Here's how the part is built. I have some questions about the finished solid (model axes, mm). Face numbers are marked on the shaded views. Coordinates: 2 decimals unless noted, no trailing zeros. Write each loop counter-clockwise with the first axis right and the second up, starting at its lowest first coordinate (ties: lowest second). Pieces come first, ordered by that corner, then holes. Notation, with made-up numbers: (64.5, -25) -> (74.5, -25) arc R28 ccw to (74.5, 8) -> close; hole circle Ø7 at (31.25, 34.25). An arc over 180 degrees is marked (long way). Use a Markdown table: item, result. Add a question column.
Item 1: If I drill on line 1 along Y through (x, z) = (0, 87); line 2 along X through (y, z) = (28.5, 110.5); line 3 along Y through (x, z) = (50, 68.5), over which ranges is the centre line in solid material (lowest first)? Write a range as from..to.
Item 2: Imagine slicing it at A-A, the plane x = 0. Write out the boundary of the cut face in (y, z) (3 decimals), and give its area (3 significant figures).
Item 3: Imagine slicing it at D-D, the plane z = 12.5. Write out the boundary of the cut face in (x, y).
Item 4: Will these pins go through, and if not, where does the flat tip stop? pin 1 Ø1.5 at (y, z) = (8.5, 82.5) entering from +X; pin 2 Ø10 at (y, z) = (50.5, 102.5) entering from +X; pin 3 Ø5 at (y, z) = (-76.5, 115.5) entering from +X.
Item 5: Imagine slicing it at C-C, the plane z = 143. Write out the boundary of the cut face in (x, y).
Item 6: If we mould it in two halves opening along X, with no side actions, what happens to the marked faces 1, 2 and 3? For each: pulls with the +X half, pulls with the -X half, needs draft (parallel to the pull), parting line crosses it, or undercut.
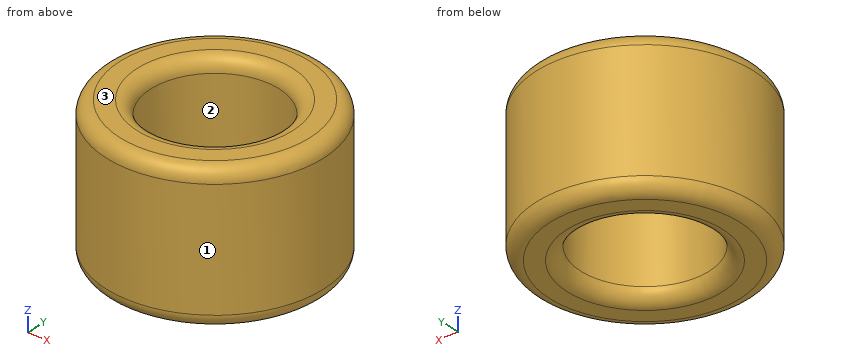
```python
from build123d import *

# Parameters (mm, degrees)
SKETCH1_R           = 127
BOSS_EXTRUDE1_DEPTH = 170
SKETCH2_R           = 75
CUT_EXTRUDE1_DEPTH  = 171
FILLET1_R           = 15.875


with BuildPart() as part:
    # Sketch1 → Boss-Extrude1 (new body)
    with BuildSketch(Plane.XY):
        Circle(SKETCH1_R)
    extrude(amount=BOSS_EXTRUDE1_DEPTH)

    # Sketch2 → Cut-Extrude1 (cut, through all)
    with BuildSketch(Plane.XY.offset(170)):
        Circle(SKETCH2_R)
    extrude(amount=-CUT_EXTRUDE1_DEPTH, mode=Mode.SUBTRACT)

    # Fillet1
    fillet1_edges = [part.edges().sort_by_distance(p)[0] for p in [
        (-127, 0, 0),
        (-127, 0, 170),
        (-75, 0, 0),
        (-75, 0, 170),
    ]]
    fillet(fillet1_edges, radius=FILLET1_R)


solid = part.part
```
Ans:
| question | item | result |
|---|---|---|
| 1 | line 1 | y = -127..-75, 75..127 |
| 1 | line 2 | x = -123.76..-69.37, 69.37..123.76 |
| 1 | line 3 | y = -116.74..-55.9, 55.9..116.74 |
| 2 | outline | (-127, 15.875) arc R15.875 ccw to (-111.125, 0) -> (-90.875, 0) arc R15.875 ccw to (-75, 15.875) -> (-75, 154.125) arc R15.875 ccw to (-90.875, 170) -> (-111.125, 170) arc R15.875 ccw to (-127, 154.125) -> close; (75, 15.875) arc R15.875 ccw to (90.875, 0) -> (111.125, 0) arc R15.875 ccw to (127, 15.875) -> (127, 154.125) arc R15.875 ccw to (111.125, 170) -> (90.875, 170) arc R15.875 ccw to (75, 154.125) -> close |
| 2 | area | 17,200 mm^2 |
| 3 | outline | circle Ø253.27 at (0, 0); hole circle Ø150.73 at (0, 0) |
| 4 | pin 1 | stops at x = 126.76 |
| 4 | pin 2 | stops at x = 118.57 |
| 4 | pin 3 | stops at x = 103.21 |
| 5 | outline | circle Ø254 at (0, 0); hole circle Ø150 at (0, 0) |
| 6 | face 1 | parting line crosses it |
| 6 | face 2 | undercut |
| 6 | face 3 | needs draft |
